from build123d import *

# Parameters (mm, degrees)
PAD_DEPTH    = 2
FILLET_R     = 1
FILLET001_R  = 1
PAD001_DEPTH = 200


with BuildPart() as part:
    # Sketch → Pad (new body)
    with BuildSketch(Plane.YZ):
        Polygon((-9.7, 0), (0, 0), (0, 12.7), (-9.7, 3), align=None)
    extrude(amount=PAD_DEPTH)

    # Fillet
    fillet_edges = [part.edges().sort_by_distance(p)[0] for p in [
        (1, 0, 12.7),
    ]]
    fillet(fillet_edges, radius=FILLET_R)

    # Fillet001
    fillet001_edges = [part.edges().sort_by_distance(p)[0] for p in [
        (1, -9.7, 3),
    ]]
    fillet(fillet001_edges, radius=FILLET001_R)

    # Sketch001 (on Face1 of Fillet001) → Pad001 (join)
    with BuildSketch(Plane(origin=(0, 0, 0), x_dir=(0, 1, 0), z_dir=(-1, 0, 0))):
        with BuildLine():
            Line((0, -3), (0, -10.285787))
            ThreePointArc((-1.707108, -10.992893), (-0.617572, -11.20905), (0, -10.285787))
            Line((-8.992894, -3.707107), (-1.707108, -10.992893))
            ThreePointArc((-8.285787, -2), (-9.209667, -2.617317), (-8.992894, -3.707107))
            Line((-8.285787, -2), (-1, -2))
            ThreePointArc((0, -3), (-0.292893, -2.292893), (-1, -2))
        make_face()
    extrude(amount=PAD001_DEPTH)


solid = part.part
Geometry: final body of the model. Coordinates: model frame, mm. A direction names the side the tool comes from. Give positions to 0.01 mm unless a question says otherwise; leave off trailing zeros. Order: outer loops, then holes, each group sorted by start corner. A loop starts at its lowest first (then second) coordinate and runs counter-clockwise, first axis right, second up. Notation, with made-up numbers: (70.5, -2) -> (75.5, -2) arc R30 cw to (75.5, 30) -> close; hole circle Ø3 at (53.25, -20.5). An arc over 180 degrees is marked (long way). Put each result on its own line as item: value.
Q1. Section A-A, the plane y = -3.5. Return loops of the section in (x, z).
Here are the results:
outline: (-200, 2) -> (0, 2) -> (0, 0) -> (2, 0) -> (2, 9.2) -> (-200, 9.2) -> close
Q2. Section B-B, the plane z = 5.5. Return loops of the section in (x, y), then the cut area to 3 significant figures.
Here are the results:
outline: (-200, -7.2) -> (2, -7.2) -> (2, 0) -> (-200, 0) -> close
area: 1,450 mm^2
Q3. Reachability of faces 1 (the face through (-98.6, -5.4, 7.3)), 2 (the face through (-99, -5, 2)) from +Z, -Z, +X, -X, +Y, -Y: full face, straight path, thin tool, end or side. Return the list, or none.
Here are the results:
face 1: +Z, +X, -X, -Y
face 2: -Z, -X, +Y, -Y
Q4. Material intervals for L1, parallel to X at y = -5.75, z = 1.25; L2, parallel to Z at x = -56, y = -0.5; L3, parallel to Y at x = -128, z = 9, sorted ascending.
Here are the results:
L1: x = 0 to 2
L2: z = 2.13 to 11.15
L3: y = -3.7 to 0
Q5. Section C-C, the plane x = -37. Return loops of the section in (y, z).
Here are the results:
outline: (-8.99, 3.71) arc R1 ccw to (-8.29, 2) -> (-1, 2) arc R1 ccw to (0, 3) -> (0, 10.29) arc R1 ccw to (-1.71, 10.99) -> close
Q6. Pin query (flat end, axial travel): pin 1 (1.5 mm diameter, centred on y = -3, z = 1.5, fed in from -X); pin 2 (3 mm diameter, centred on x = -59, y = -2.5, fed in from -Z); pin 3 (5 mm diameter, centred on x = -26, z = 7, fed in from -Y); pin 4 (2 mm diameter, centred on y = -6.5, z = 8, fed in from +X). Return the tip coordinate at first contact, or that it passes through.
Here are the results:
pin 1: stops at x = -200
pin 2: stops at z = 2
pin 3: stops at y = -8.2
pin 4: passes through
